from build123d import *

# Parameters (mm, degrees)
EXTRUDE_1_DEPTH      = 20
SKETCH_4_R           = 6.5
SKETCH_4_R_2         = 3
EXTRUDE_2_DEPTH      = 1.7
SKETCH_5_R           = 3
EXTRUDE_3_DEPTH      = 2.7
SKETCH_6_R           = 3.2
EXTRUDE_4_DEPTH      = 3
SKETCH_7_R           = 1
CUT_EXTRUDE_41_DEPTH = 5.7
SKETCH_8_R           = 6.5
SKETCH_8_R_2         = 3.5
EXTRUDE_5_DEPTH      = 1.7
SKETCH_9_R           = 2.5
EXTRUDE_6_DEPTH      = 3
SKETCH_10_R          = 1
CUT_EXTRUDE_42_DEPTH = 5


with BuildPart() as part:
    # 草图1 → 凸台-拉伸1 (new body)
    with BuildSketch(Plane(origin=(0, 0, 0), x_dir=(1, 0, 0), z_dir=(0, 1, 0))):
        Polygon((-57.643399256, 26.149695183), (-19.643399256, 26.149695183), (-18.643399256, 25.149695183), (-18.643399256, -12.850304817), (-19.643399256, -13.850304817), (-57.643399256, -13.850304817), (-58.643399256, -12.850304817), (-58.643399256, 25.149695183), align=None)
    extrude(amount=EXTRUDE_1_DEPTH)

    # 草图4 → 凸台-拉伸2 (add)
    with BuildSketch(Plane(origin=(0, 0, -26.149695183), x_dir=(-1, 0, 0), z_dir=(0, 0, -1))):
        with Locations((49.643399256, 10)):
            Circle(SKETCH_4_R)
        with Locations((49.643399256, 10)):
            Circle(SKETCH_4_R_2, mode=Mode.SUBTRACT)
    extrude(amount=EXTRUDE_2_DEPTH)

    # 草图5 → 凸台-拉伸3 (add)
    with BuildSketch(Plane(origin=(0, 0, -26.149695183), x_dir=(-1, 0, 0), z_dir=(0, 0, -1))):
        with Locations((49.643399256, 10)):
            Circle(SKETCH_5_R)
    extrude(amount=EXTRUDE_3_DEPTH)

    # 草图6 → 凸台-拉伸4 (add)
    with BuildSketch(Plane(origin=(0, 0, -28.849695183), x_dir=(-1, 0, 0), z_dir=(0, 0, -1))):
        with Locations((49.643399256, 10)):
            Circle(SKETCH_6_R)
    extrude(amount=EXTRUDE_4_DEPTH)

    # 草图7 → 切除-拉伸41 (cut)
    with BuildSketch(Plane(origin=(0, 0, -31.849695183), x_dir=(-1, 0, 0), z_dir=(0, 0, -1))):
        with Locations((49.643399256, 10)):
            Circle(SKETCH_7_R)
    extrude(amount=-CUT_EXTRUDE_41_DEPTH, mode=Mode.SUBTRACT)

    # 草图8 → 凸台-拉伸5 (add)
    with BuildSketch(Plane.XY.offset(13.850304817)):
        with Locations((-49.643399256, 10)):
            Circle(SKETCH_8_R)
        with Locations((-49.643399256, 10)):
            Circle(SKETCH_8_R_2, mode=Mode.SUBTRACT)
    extrude(amount=EXTRUDE_5_DEPTH)

    # 草图9 → 凸台-拉伸6 (add)
    with BuildSketch(Plane.XY.offset(13.850304817)):
        with Locations((-49.643399256, 10)):
            Circle(SKETCH_9_R)
    extrude(amount=EXTRUDE_6_DEPTH)

    # 草图10 → 切除-拉伸42 (cut)
    with BuildSketch(Plane.XY.offset(16.850304817)):
        with Locations((-49.643399256, 10)):
            Circle(SKETCH_10_R)
    extrude(amount=-CUT_EXTRUDE_42_DEPTH, mode=Mode.SUBTRACT)


solid = part.part
Can you work these out from the model? Positions are in its coordinate system, mm. A direction names the side the tool comes from. Give positions to 0.01 mm unless a question says otherwise; leave off trailing zeros. Loops run counter-clockwise (first coordinate to the right, second up) from the corner with the lowest first, then second, coordinate; pieces in that order, holes last. Notation, with made-up numbers: M 55,45 L 70,45 A31 cw 70,78 Z; hole C -23,12.25 d3. An arc over 180 degrees is marked long. One line per item, written item: value. Start each with the question number.
1) If we section it at A-A, the plane y = 1.5: Write out the boundary of the cut face in (x, z).
2) If we section it at B-B, the plane x = -51.5: Write out the boundary of the cut face in (y, z), and give its area (3 significant figures).
3) If we section it at D-D, the plane x = -25.5: Write out the boundary of the cut face in (y, z).
4) If we section it at C-C, the plane y = 14.5: Write out the boundary of the cut face in (x, z), and give its area (3 significant figures).
5) I'm going to push flat-ended pins straight in: pin 1 (10 mm diameter, centred on x = -33.5, y = 10, fed in from +Z); pin 2 (3 mm diameter, centred on x = -53.5, y = 8.5, fed in from +Z); pin 3 (4 mm diameter, centred on x = -33, y = 14, fed in from -Z). Where does each tip first touch, or does it pass through?
6) On a 3-axis mill with a long thin cutter (end or side, diameter ignored), from which of +Z, -Z, +X, -X, +Y, -Y can I reach the whole of each face in a straight line? I mean faces 4 (the face through (-43.15, 10.29, -26.99)), 5 (the face through (-48.69, 10.3, 14.39)), 6 (the face through (-46.646, 10.132, -28.343)), 7 (the face through (-58.15, 9.86, -25.643)). Say none if no direction works.
7) Thinking about a two-plate mould opening in X: for faces 1 (the face through (-38, 0, -6)), 2 (the face through (-58.136, 9.86, 13.357)), 3 (the face through (-51.63, 8.48, 15.33)), which applies, +X half, -X half, draft (parallel to the pull), parting line (faces both ways), or undercut?
8) If I drill on line 1 (Z direction, x = -30, y = 13.25); line 2 (Z direction, x = -55, y = 10.75), over which ranges is the centre line in solid material (lowest first)? Write a range as [from, to].
Completed:
1. outline: M -58.64,-25.15 L -57.64,-26.15 L -19.64,-26.15 L -18.64,-25.15 L -18.64,12.85 L -19.64,13.85 L -57.64,13.85 L -58.64,12.85 Z
2. outline: M 0,-26.15 L 3.77,-26.15 L 3.77,-27.85 L 7.64,-27.85 L 7.64,-28.85 L 7.39,-28.85 L 7.39,-31.85 L 12.61,-31.85 L 12.61,-28.85 L 12.36,-28.85 L 12.36,-27.85 L 16.23,-27.85 L 16.23,-26.15 L 20,-26.15 L 20,13.85 L 16.23,13.85 L 16.23,15.55 L 12.97,15.55 L 12.97,13.85 L 11.67,13.85 L 11.67,16.85 L 8.33,16.85 L 8.33,13.85 L 7.03,13.85 L 7.03,15.55 L 3.77,15.55 L 3.77,13.85 L 0,13.85 Z
2. area: 863 mm^2
3. outline: M 0,-26.15 L 20,-26.15 L 20,13.85 L 0,13.85 Z
4. outline: M -58.64,-25.15 L -57.64,-26.15 L -54.33,-26.15 L -54.33,-27.85 L -44.95,-27.85 L -44.95,-26.15 L -19.64,-26.15 L -18.64,-25.15 L -18.64,12.85 L -19.64,13.85 L -44.95,13.85 L -44.95,15.55 L -54.33,15.55 L -54.33,13.85 L -57.64,13.85 L -58.64,12.85 Z
4. area: 1,630 mm^2
5. pin 1: stops at z = 13.85
5. pin 2: stops at z = 15.55
5. pin 3: stops at z = -26.15
6. face 4: -Z
6. face 5: +Z
6. face 6: none
6. face 7: -Z, -X, +Y, -Y
7. face 1: draft
7. face 2: -X half
7. face 3: undercut
8. line 1: z = [-26.15, 13.85]
8. line 2: z = [-27.85, 15.55]
